```python
from build123d import *

# Parameters (mm, degrees)
F0_W     = 1028.7
F0_H     = 1028.7
F1_DEPTH = 12.7
F2_W     = 1028.7
F2_H     = 1028.7
F2_W_2   = 1003.3
F2_H_2   = 1003.3
F3_DEPTH = 584.2
F4_W     = 1028.7
F4_H     = 1028.7
F5_DEPTH = 12.7
F6_W     = 501.65
F6_H     = 488.95
F7_DEPTH = 152.4
F9_DEPTH = 12.7


with BuildPart() as f1:
    # F0 (on Top) → F1 (new body)
    with BuildSketch(Plane.XY):
        with Locations((514.35, 514.35)):
            Rectangle(F0_W, F0_H)
    extrude(amount=F1_DEPTH)

    # F2 (on Top) → F3 (join)
    with BuildSketch(Plane.XY):
        with Locations((514.35, 514.35)):
            Rectangle(F2_W, F2_H)
        with Locations((514.35, 514.35)):
            Rectangle(F2_W_2, F2_H_2, mode=Mode.SUBTRACT)
    extrude(amount=F3_DEPTH)

    # F4 (on face) → F5 (join)
    with BuildSketch(Plane.XY.offset(584.2)):
        with Locations((514.35, 514.35)):
            Rectangle(F4_W, F4_H)
    extrude(amount=F5_DEPTH)

    # F6 (on face) → F7 (join)
    with BuildSketch(Plane.XY.offset(596.9)):
        Polygon((1028.7, 1028.7), (0, 1028.7), (0, 0), (12.7, 0), (12.7, 12.7), (12.7, 514.35), (514.35, 514.35), (514.35, 12.7), (514.35, 0), (527.05, 0), (527.05, 12.7), (527.05, 514.35), (952.5, 514.35), (1028.7, 514.35), (1028.7, 527.05), (952.5, 527.05), (527.05, 527.05), (527.05, 1016), (1016, 1016), (1028.7, 1016), align=None)
        with Locations((263.525, 771.525)):
            Rectangle(F6_W, F6_H, mode=Mode.SUBTRACT)
    extrude(amount=F7_DEPTH)

    # F8 (on face) → F9 (join)
    with BuildSketch(Plane.XY.offset(749.3)):
        Polygon((0, 1028.7), (0, 0), (527.05, 0), (1028.7, 514.35), (1028.7, 1028.7), align=None)
    extrude(amount=F9_DEPTH)


solid = f1.part
```
The listing builds one solid part. Answer for the finished solid, in the listing's coordinates (mm). A direction names the side the tool comes from. Coordinates: 2 decimals unless noted, no trailing zeros. Write each loop counter-clockwise with the first axis right and the second up, starting at its lowest first coordinate (ties: lowest second). Pieces come first, ordered by that corner, then holes.
Q1. Section C-C, the plane y = 642 is taken. Write down the section's boundary in (x, z), then the cut area to 3 significant figures.
Returned:
outline: (0, 0) - (1028.7, 0) - (1028.7, 596.9) - (527.05, 596.9) - (527.05, 749.3) - (1028.7, 749.3) - (1028.7, 762) - (0, 762) - close; hole (12.7, 12.7) - (1016, 12.7) - (1016, 584.2) - (12.7, 584.2) - close; hole (12.7, 596.9) - (514.35, 596.9) - (514.35, 749.3) - (12.7, 749.3) - close
area: 57,600 mm2
Q2. The mould has two halves that part along Y. Classify faces 1 (the flat face through (774, 261, 596.9)), 2 (the flat face through (774.36, 253.57, 755.56)), 3 (the flat face through (507, 521, 584.2)): released by +Y, released by -Y, zero draft, split by the parting line, or undercut.
Returned:
face 1: zero draft
face 2: released by -Y
face 3: undercut
Q3. Section A-A, the plane z = 232.5 is taken. Write down the section's boundary in (x, y), then the cut area to 3 significant figures.
Returned:
outline: (0, 0) - (1028.7, 0) - (1028.7, 1028.7) - (0, 1028.7) - close; hole (12.7, 12.7) - (1016, 12.7) - (1016, 1016) - (12.7, 1016) - close
area: 51,600 mm2
Q4. Which of the six approach directions +Z, -Z, +X, -X, +Y, -Y give full straight-line access (tool end or side, diameter ignored) to faces 4 (the flat face through (260, 514.35, 672)), 5 (the flat face through (719, 318, 749.3)), 6 (the flat face through (12.7, 507, 294)), 7 (the flat face through (774, 775, 749.3))?
Returned:
face 4: -Y
face 5: +X, -Y
face 6: none
face 7: +X
Q5. Section B-B, the plane x = 221.5 is taken. Write down the section's boundary in (y, z), then the cut area to 3 significant figures.
Returned:
outline: (0, 0) - (1028.7, 0) - (1028.7, 762) - (0, 762) - (0, 749.3) - (514.35, 749.3) - (514.35, 596.9) - (0, 596.9) - close; hole (12.7, 12.7) - (1016, 12.7) - (1016, 584.2) - (12.7, 584.2) - close; hole (527.05, 596.9) - (1016, 596.9) - (1016, 749.3) - (527.05, 749.3) - close
area: 57,600 mm2
Q6. Find the intervals of material crossed by line 1 along Z through (x, y) = (82, 657); line 2 along Z through (x, y) = (797, 206); line 3 along X through (y, z) = (426, 454), in increasing order.
Returned:
line 1: z = 0 to 12.7, 584.2 to 596.9, 749.3 to 762
line 2: z = 0 to 12.7, 584.2 to 596.9
line 3: x = 0 to 12.7, 1016 to 1028.7
Q7. Given P1, Ø8, axis at x = 788, z = 333, coming from the -Y side, flat-ended and moving along its own axis, determine where the tip first touches the part or whether it passes through.
Returned:
P1: stops at y = 0
